from build123d import *

# Parameters (mm, degrees)
ESBO_O2_R                = 0.75
RESSALTO_EXTRUS_O1_DEPTH = 2
PADR_OCIRCULAR1_COUNT    = 4
ESBO_O3_R                = 4
ESBO_O3_R_2              = 2.5
RESSALTO_EXTRUS_O2_DEPTH = 3.5
CORTE_EXTRUS_O1_START    = -1
ESBO_O4_R                = 2.5
ESBO_O4_R_2              = 0.75
CORTE_EXTRUS_O1_DEPTH    = 1
RESSALTO_EXTRUS_O3_START = 1
ESBO_O5_R                = 3
ESBO_O5_R_2              = 2.5
RESSALTO_EXTRUS_O3_DEPTH = 1


with BuildPart() as part:
    # Esboço2 → Ressalto-extrusão1 (new body)
    with BuildSketch(Plane(origin=(0, 0, 0), x_dir=(1, 0, 0), z_dir=(0, 1, 0))):
        with BuildLine():
            Line((-10.270723649, 1.981592467), (-4.128356106, 2.82075803))
            ThreePointArc((-4.128356106, 2.82075803), (-2.520023904, 4.318504316), (-0.424825461, 4.981919643))
            ThreePointArc((-0.424825461, 4.981919643), (0, 4.85), (0.424825461, 4.981919643))
            ThreePointArc((0.424825461, 4.981919643), (3.535533906, 3.535533906), (4.981919643, 0.424825461))
            ThreePointArc((4.981919643, 0.424825461), (4.85, 0), (4.981919643, -0.424825461))
            ThreePointArc((4.981919643, -0.424825461), (3.535533906, -3.535533906), (0.424825461, -4.981919643))
            ThreePointArc((0.424825461, -4.981919643), (0, -4.85), (-0.424825461, -4.981919643))
            ThreePointArc((-0.424825461, -4.981919643), (-2.520023904, -4.318504316), (-4.128356106, -2.82075803))
            Line((-4.128356106, -2.82075803), (-10.270723649, -1.981592467))
            ThreePointArc((-10.270723649, -1.981592467), (-12, 0), (-10.270723649, 1.981592467))
        make_face()
        with Locations(Location((0, 0, 0), (0, 0, 270))):
            Circle(ESBO_O2_R, mode=Mode.SUBTRACT)
        with Locations(Location((-5.6, 0, 0), (0, 0, 270))):
            Circle(ESBO_O2_R, mode=Mode.SUBTRACT)
        with Locations(Location((-7.8, 0, 0), (0, 0, 270))):
            Circle(ESBO_O2_R, mode=Mode.SUBTRACT)
        with Locations(Location((-10, 0, 0), (0, 0, 270))):
            Circle(ESBO_O2_R, mode=Mode.SUBTRACT)
    ressalto_extrus_o1 = extrude(amount=RESSALTO_EXTRUS_O1_DEPTH)

    # PadrãoCircular1: Ressalto-extrusão1 ×4 about axis
    padr_ocircular1_axis = Axis((0, 0, 0), (0, 1, 0))
    for i in range(1, PADR_OCIRCULAR1_COUNT):
        add(ressalto_extrus_o1.rotate(padr_ocircular1_axis, i * 360 / PADR_OCIRCULAR1_COUNT))

    # Esboço3 → Ressalto-extrusão2 (add)
    with BuildSketch(Plane(origin=(0, 2, 0), x_dir=(1, 0, 0), z_dir=(0, 1, 0))):
        with Locations(Location((0, 0, 0), (0, 0, 270))):
            Circle(ESBO_O3_R)
        with Locations(Location((0, 0, 0), (0, 0, 270))):
            Circle(ESBO_O3_R_2, mode=Mode.SUBTRACT)
    extrude(amount=RESSALTO_EXTRUS_O2_DEPTH)

    # Esboço4 → Corte-extrusão1 (cut)
    with BuildSketch(Plane(origin=(0, 2, 0), x_dir=(1, 0, 0), z_dir=(0, 1, 0)).offset(CORTE_EXTRUS_O1_START)):
        with Locations(Location((0, 0, 0), (0, 0, 270))):
            Circle(ESBO_O4_R)
        with Locations(Location((0, 0, 0), (0, 0, 270))):
            Circle(ESBO_O4_R_2, mode=Mode.SUBTRACT)
    extrude(amount=CORTE_EXTRUS_O1_DEPTH, mode=Mode.SUBTRACT)

    # Esboço5 → Ressalto-extrusão3 (add)
    with BuildSketch(Plane.XZ.offset(RESSALTO_EXTRUS_O3_START)):
        with Locations(Location((0, 0, 0), (0, 0, 90))):
            Circle(ESBO_O5_R)
        with Locations(Location((0, 0, 0), (0, 0, 90))):
            Circle(ESBO_O5_R_2, mode=Mode.SUBTRACT)
    extrude(amount=-RESSALTO_EXTRUS_O3_DEPTH)


solid = part.part
Model file for the job. Use its own axes, mm. A direction names the side the tool comes from. Give positions to 0.01 mm unless a question says otherwise; leave off trailing zeros. Order: outer loops, then holes, each group sorted by start corner. A loop starts at its lowest first (then second) coordinate and runs counter-clockwise, first axis right, second up. Notation, with made-up numbers: (-32, 51.25) - (-17, 51.25) arc R23 cw to (-17, 64.25) - close; hole circle Ø11 at (2.25, 55). An arc over 180 degrees is marked (long way). One line per item, written item: value.
Item 1: Two-plate mould, pull along X, no slides. Class faces 3 (the cylindrical face through (-0.9, -0.51, 2.86)), 4 (the cylindrical face through (-3.53, 0.99, 3.54)), 5 (the cylindrical face through (7.056, 0.986, 0.098)), 6 (the cylindrical face through (2.44, -0.51, -0.54)): released by +X, released by -X, zero draft, split by the parting line, or undercut.
Response values:
face 3: split by the parting line
face 4: released by -X
face 5: undercut
face 6: undercut
Item 2: Slice it at B-B (x = 7.8). List the corners of the cut face in (y, z), then the cut area to 3 significant figures.
Response values:
outline: (0, -2.32) - (2, -2.32) - (2, -0.75) - (0, -0.75) - close; (0, 0.75) - (2, 0.75) - (2, 2.32) - (0, 2.32) - close
area: 6.28 mm2
Item 3: Slice it at A-A (y = 1.5). Give the number of separate pieces and of enclosed holes in the cut face, then the cut area to 3 significant figures.
Response values:
separate pieces: 1
enclosed holes: 13
area: 163 mm2
Item 4: Slice it at C-C (z = 7.8). List the corners of the cut face in (x, y), then the cut area to 3 significant figures.
Response values:
outline: (-2.32, 0) - (-0.75, 0) - (-0.75, 2) - (-2.32, 2) - close; (0.75, 0) - (2.32, 0) - (2.32, 2) - (0.75, 2) - close
area: 6.28 mm2
Item 5: Wall check: line 1 (X direction, y = 1.5, z = 8); line 2 (Y direction, x = 0.75, z = 4.75); line 3 (Z direction, x = 5.5, y = 0.5). Give the ranges that are in metal, low to high.
Response values:
line 1: -2.29 to -0.72, 0.72 to 2.29
line 2: 0 to 2
line 3: -2.63 to -0.74, 0.74 to 2.63
Item 6: Pin check, flat tips, straight feed: pin 1 Ø1.7 at (x, z) = (-7.8, 0) entering from -Y; pin 2 Ø1.5 at (x, z) = (1, -7.5) entering from +Y; pin 3 Ø3 at (x, y) = (0, 5) entering from +Z. Stop position of each tip, or through.
Response values:
pin 1: y = 0
pin 2: y = 2
pin 3: z = 4
Item 7: Tool access for faces 1 (the flat face through (-2, -1, -2)), 2 (the cylindrical face through (-2.44, 3.22, -0.54)): list every direction of +Z, -Z, +X, -X, +Y, -Y with a clear straight run to the whole face (end or side of a thin tool).
Response values:
face 1: +Z, -Z, +X, -X, -Y
face 2: +Y
